from build123d import *

# Parameters (mm, degrees)
SKETCH1_W                    = 380
SKETCH1_H                    = 200
BASE_FLANGE1_DEPTH           = 4
EDGE_FLANGE1_STRIP_W         = 17.4732
EDGE_FLANGE1_STRIP_H         = 4
EDGE_FLANGE1_STRIP_CUT_DEPTH = 380
EDGE_FLANGE1_DEPTH           = 380
EDGE_FLANGE2_STRIP_W         = 17.4732
EDGE_FLANGE2_STRIP_H         = 4
EDGE_FLANGE2_STRIP_CUT_DEPTH = 199.2634
EDGE_FLANGE2_DEPTH           = 199.2634
EDGE_FLANGE3_STRIP_W         = 17.4732
EDGE_FLANGE3_STRIP_H         = 4
EDGE_FLANGE3_STRIP_CUT_DEPTH = 199.2634
EDGE_FLANGE3_DEPTH           = 199.2634
EXTRUDE1_DEPTH               = 583.765819176
EXTRUDE2_DEPTH               = 583.765819176
FILLET1_R                    = 2
SKETCH15_W                   = 23.472504697
SKETCH15_H                   = 33.276719244
EXTRUDE6_DEPTH               = 10
SKETCH16_W                   = 26.053110818
SKETCH16_H                   = 17.698317339
EXTRUDE7_DEPTH               = 10
FILLET2_R                    = 2
SKETCH17_W                   = 318
SKETCH17_H                   = 161.8
EXTRUDE8_DEPTH               = 578.470345559
FILLET3_R                    = 20
SKETCH18_R                   = 3
EXTRUDE9_DEPTH               = 578.470345559
LPATTERN1_COUNT              = 17
LPATTERN1_PITCH              = 10
SKETCH20_W                   = 800
SKETCH20_H                   = 800
EXTRUDE15_DEPTH              = 581.110334333
FILLET4_R                    = 20
FILLET5_R                    = 2
FILLET6_R                    = 2


# Sheet-metal steps are written as plain solids
with BuildPart() as part:
    # Sketch1 → Base-Flange1 (new body)
    with BuildSketch(Plane.XY):
        with Locations((190, 100)):
            Rectangle(SKETCH1_W, SKETCH1_H)
    extrude(amount=BASE_FLANGE1_DEPTH)

    # Edge-Flange1 strip (across the edge) → Edge-Flange1 strip cut (cut)
    with BuildSketch(Plane(origin=(380, 200, 4), x_dir=(0, -1, 0), z_dir=(-1, 0, 0))):
        with Locations((-8, -2)):
            Rectangle(EDGE_FLANGE1_STRIP_W, EDGE_FLANGE1_STRIP_H)
    extrude(amount=EDGE_FLANGE1_STRIP_CUT_DEPTH, mode=Mode.SUBTRACT)

    # Edge-Flange1 section (across the edge) → Edge-Flange1 (add)
    with BuildSketch(Plane(origin=(380, 200, 4), x_dir=(0, -1, 0), z_dir=(-1, 0, 0))):
        with BuildLine():
            Line((-4, 0.7366), (-4, 10))
            Line((-4, 10), (0, 10))
            Line((0, 10), (0, 0.7366))
            ThreePointArc((0, 0.7366), (0.215745145, 0.215745145), (0.7366, 0))
            Line((0.7366, 0), (0.7366, -4))
            ThreePointArc((0.7366, -4), (-2.61268198, -2.61268198), (-4, 0.7366))
        make_face()
    extrude(amount=EDGE_FLANGE1_DEPTH)

    # Edge-Flange2 strip (across the edge) → Edge-Flange2 strip cut (cut)
    with BuildSketch(Plane(origin=(0, 199.2634, 4), x_dir=(1, 0, 0), z_dir=(0, -1, 0))):
        with Locations((-8, -2)):
            Rectangle(EDGE_FLANGE2_STRIP_W, EDGE_FLANGE2_STRIP_H)
    extrude(amount=EDGE_FLANGE2_STRIP_CUT_DEPTH, mode=Mode.SUBTRACT)

    # Edge-Flange2 section (across the edge) → Edge-Flange2 (add)
    with BuildSketch(Plane(origin=(0, 199.2634, 4), x_dir=(1, 0, 0), z_dir=(0, -1, 0))):
        with BuildLine():
            Line((-4, 0.7366), (-4, 380))
            Line((-4, 380), (0, 380))
            Line((0, 380), (0, 0.7366))
            ThreePointArc((0, 0.7366), (0.215745145, 0.215745145), (0.7366, 0))
            Line((0.7366, 0), (0.7366, -4))
            ThreePointArc((0.7366, -4), (-2.61268198, -2.61268198), (-4, 0.7366))
        make_face()
    extrude(amount=EDGE_FLANGE2_DEPTH)

    # Edge-Flange3 strip (across the edge) → Edge-Flange3 strip cut (cut)
    with BuildSketch(Plane(origin=(380, 0, 4), x_dir=(-1, 0, 0), z_dir=(0, 1, 0))):
        with Locations((-8, -2)):
            Rectangle(EDGE_FLANGE3_STRIP_W, EDGE_FLANGE3_STRIP_H)
    extrude(amount=EDGE_FLANGE3_STRIP_CUT_DEPTH, mode=Mode.SUBTRACT)

    # Edge-Flange3 section (across the edge) → Edge-Flange3 (add)
    with BuildSketch(Plane(origin=(380, 0, 4), x_dir=(-1, 0, 0), z_dir=(0, 1, 0))):
        with BuildLine():
            Line((-4, 0.7366), (-4, 380))
            Line((-4, 380), (0, 380))
            Line((0, 380), (0, 0.7366))
            ThreePointArc((0, 0.7366), (0.215745145, 0.215745145), (0.7366, 0))
            Line((0.7366, 0), (0.7366, -4))
            ThreePointArc((0.7366, -4), (-2.61268198, -2.61268198), (-4, 0.7366))
        make_face()
    extrude(amount=EDGE_FLANGE3_DEPTH)

    # Sketch12 → Extrude1 (cut, through all)
    with BuildSketch(Plane.ZY.offset(4)):
        with BuildLine():
            ThreePointArc((384, 179.2634), (179.031265067, 127.81319162), (10.7366, 0))
            Line((10.7366, 0), (384, 0))
            Line((384, 0), (384, 179.2634))
        make_face()
    extrude(amount=-EXTRUDE1_DEPTH, mode=Mode.SUBTRACT)

    # Sketch13 → Extrude2 (cut, through all)
    with BuildSketch(Plane.ZY.offset(4)):
        Polygon((14.85780282, 191.8), (38.9966, 191.8), (38.9966, 197.8), (42.9966, 197.8), (42.9966, 191.8), (328.9966, 191.8), (328.9966, 197.8), (332.9966, 197.8), (332.9966, 191.8), (384, 191.8), (384, 199.2634), (4.7366, 199.2634), (4.7366, 191.8), align=None)
    extrude(amount=-EXTRUDE2_DEPTH, mode=Mode.SUBTRACT)

    # Fillet1
    fillet1_edges = [part.edges().sort_by_distance(p)[0] for p in [
        (382, 197.8, 38.9966),
        (382, 197.8, 42.9966),
        (382, 197.8, 328.9966),
        (382, 197.8, 332.9966),
        (-2, 197.8, 328.9966),
        (-2, 197.8, 332.9966),
        (-2, 197.8, 42.9966),
        (-2, 197.8, 38.9966),
    ]]
    fillet(fillet1_edges, radius=FILLET1_R - 0.0001)  # a hair under: the kernel refuses the full size

    # Sketch15 → Extrude6 (cut)
    with BuildSketch(Plane.ZY.offset(4)):
        with Locations((8.784947937, 208.438359622)):
            Rectangle(SKETCH15_W, SKETCH15_H)
    extrude(amount=-EXTRUDE6_DEPTH, mode=Mode.SUBTRACT)

    # Sketch16 → Extrude7 (cut)
    with BuildSketch(Plane(origin=(384, 0, 0), x_dir=(0, 0, -1), z_dir=(1, 0, 0))):
        with Locations((-6.110925327, 200.64915867)):
            Rectangle(SKETCH16_W, SKETCH16_H)
    extrude(amount=-EXTRUDE7_DEPTH, mode=Mode.SUBTRACT)

    # Fillet2
    fillet2_edges = [part.edges().sort_by_distance(p)[0] for p in [
        (6, 202, 14),
        (374, 202, 14),
    ]]
    fillet(fillet2_edges, radius=FILLET2_R)

    # Sketch17 → Extrude8 (cut, through all)
    with BuildSketch(Plane.XY.offset(4)):
        with Locations((190, 80.9)):
            Rectangle(SKETCH17_W, SKETCH17_H)
    extrude(amount=-EXTRUDE8_DEPTH, mode=Mode.SUBTRACT)

    # Fillet3
    fillet3_edges = [part.edges().sort_by_distance(p)[0] for p in [
        (31, 161.8, 2),
        (349, 161.8, 2),
    ]]
    fillet(fillet3_edges, radius=FILLET3_R)

    # Sketch18 → Extrude9 (cut, through all)
    with BuildSketch(Plane.XY.offset(4)):
        with Locations((15, 175)):
            Circle(SKETCH18_R)
        with Locations((365, 175)):
            Circle(SKETCH18_R)
    extrude9 = extrude(amount=-EXTRUDE9_DEPTH, mode=Mode.SUBTRACT)

    # LPattern1: Extrude9 ×17
    with Locations(*[(0, -i * LPATTERN1_PITCH, 0) for i in range(1, LPATTERN1_COUNT)]):
        add(extrude9, mode=Mode.SUBTRACT)

    # Sketch20 → Extrude15 (cut, through all)
    with BuildSketch(Plane(origin=(0, 0, 0), x_dir=(-1, 0, 0), z_dir=(0, 0, -1))):
        with Locations((115, -121.057151892)):
            Rectangle(SKETCH20_W, SKETCH20_H)
    extrude(amount=-EXTRUDE15_DEPTH, mode=Mode.SUBTRACT)

    # Fillet4
    fillet4_edges = [part.edges().sort_by_distance(p)[0] for p in [
        (285, 161.8, 2),
    ]]
    fillet(fillet4_edges, radius=FILLET4_R)

    # Fillet5
    fillet5_edges = [part.edges().sort_by_distance(p)[0] for p in [
        (285, 202, 14),
    ]]
    fillet(fillet5_edges, radius=FILLET5_R)

    # Fillet6
    fillet6_edges = [part.edges().sort_by_distance(p)[0] for p in [
        (382, 179.2634, 384),
        (382, 191.8, 384),
    ]]
    fillet(fillet6_edges, radius=FILLET6_R)


solid = part.part
Geometry check sheet. Reference: the model listing, model coordinates, mm. A direction names the side the tool comes from. Coordinates: 2 decimals unless noted, no trailing zeros. Order: outer loops, then holes, each group sorted by start corner. A loop starts at its lowest first (then second) coordinate and runs counter-clockwise, first axis right, second up. Notation, with made-up numbers: (-9.75, 81) - (32.25, 81) arc R18 cw to (32.25, 103) - close; hole circle Ø7 at (55, 79.5). An arc over 180 degrees is marked (long way). Answer in a Markdown table with one row per item. Add a question column.
1) Cross-section at B-B, the plane z = 76.5. Record the cut outline in (x, y), then the cut area to 3 significant figures.
2) Gauge pin test, flat ends, axial feed: P1, Ø9.5, axis at x = 365, y = 45, coming from the +Z side; P2, Ø4.5, axis at x = 381, y = 195, coming from the +Z side; P3, Ø4.5, axis at x = 382.5, y = 193, coming from the -Z side. Record the tip position at first contact, or that the pin passes through.
3) Cross-section at C-C, the plane z = 123. Record the cut outline in (x, y), then the cut area to 3 significant figures.
4) Release check for a two-part mould opening along Y. For faces 1 (the cylindrical face through (291.014, 167.503, 1.972)), 2 (the flat face through (374, 199, 3)), 3 (the flat face through (330, 204, 9)) record: +Y half, -Y half, draft (parallel to the pull), parting line (faces both ways), or undercut.
5) Set-up check for faces 4 (the flat face through (380, 141, 113)), 5 (the cylindrical face through (343.297, 155.786, 1.972)), 6 (the flat face through (381, 191.8, 19)), 7 (the flat face through (352, 123, 4)), 8 (the flat face through (330, 200, 9)): record each of +Z, -Z, +X, -X, +Y, -Y from which the full face is reachable in a straight line by a thin tool's end or side.
6) Cross-section at A-A, the plane x = 314.5. Record the cut outline in (y, z), then the cut area to 3 significant figures.
7) Material ranges on line 1 along Z through (x, y) = (353, 27.5); line 2 along X through (y, z) = (188, 21.5), recorded low to high. Write a range as [from, to].
Check result:
| question | item | result |
|---|---|---|
| 1 | outline | (380, 63.11) - (384, 63.11) - (384, 191.8) - (380, 191.8) - close |
| 1 | area | 515 mm² |
| 2 | P1 | stops at z = 4 |
| 2 | P2 | stops at z = 333 |
| 2 | P3 | stops at z = 0.19 |
| 3 | outline | (380, 96.57) - (384, 96.57) - (384, 191.8) - (380, 191.8) - close |
| 3 | area | 381 mm² |
| 4 | face 1 | -Y half |
| 4 | face 2 | draft |
| 4 | face 3 | +Y half |
| 5 | face 4 | +Z, -X, +Y, -Y |
| 5 | face 5 | +Z, -Z, -X, -Y |
| 5 | face 6 | -Z, +X, +Y |
| 5 | face 7 | +Z, -X, -Y |
| 5 | face 8 | +Z, +X, -X, -Y |
| 6 | outline | (161.8, 0) - (199.26, 0) arc R4.74 ccw to (204, 4.74) - (204, 14) - (200, 14) - (200, 4.74) arc R0.74 cw to (199.26, 4) - (161.8, 4) - close |
| 6 | area | 204 mm² |
| 7 | line 1 | z = [0, 4] |
| 7 | line 2 | x = [380, 384] |
